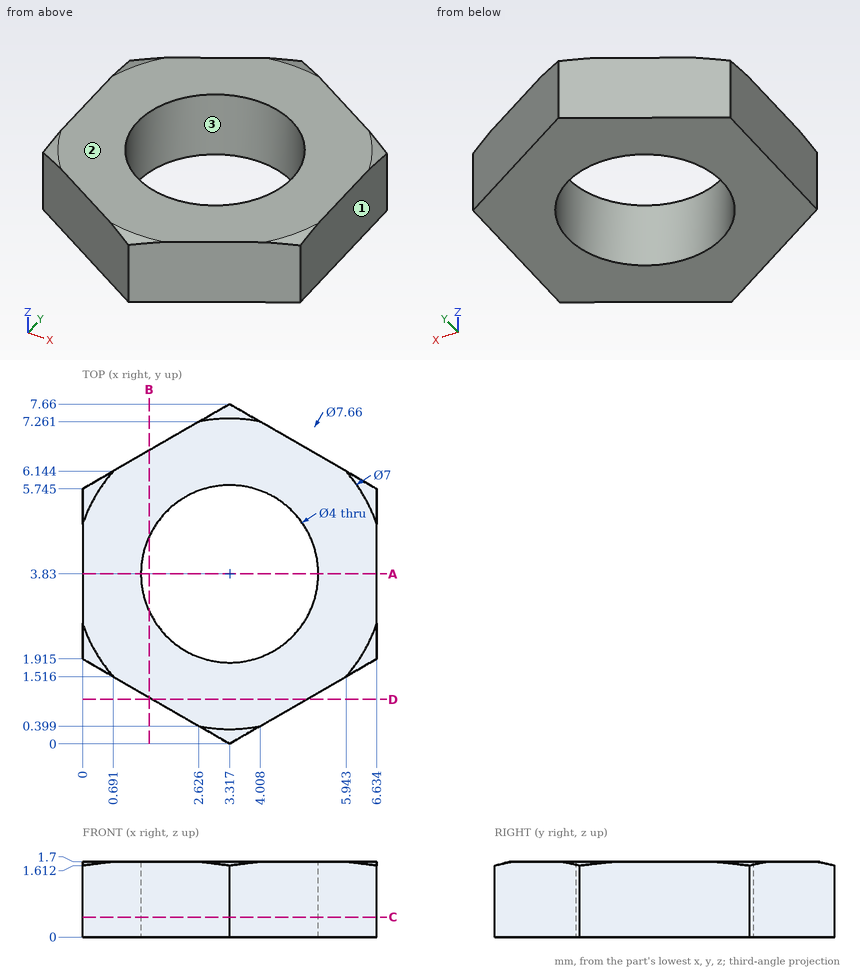
Part print with two shaded views. Sizes in mm from the minimum x, y, z corner. Round coordinates to 2 decimals unless told otherwise and drop trailing zeros. Write each loop counter-clockwise with the first axis right and the second up, starting at its lowest first coordinate (ties: lowest second). Pieces come first, ordered by that corner, then holes. Notation, with made-up numbers: M -12,-38 L 16,-38 A20 cw 16,-31 Z; hole C 43,24.25 d9. An arc over 180 degrees is marked long. Use CSV: the item, a comma, the result in double quotes.
1. Two-plate mould, pull along X, no slides. Class the marked faces 1, 2 and 3: +X half, -X half, draft (parallel to the pull), parting line (faces both ways), or undercut.
Reply:
face 1,"+X half"
face 2,"draft"
face 3,"undercut"
2. Flat gauge pin, fed straight in: pin 1 (3 mm diameter, centred on x = 3.32, y = 3.83, fed in from +Z). Where does the tip first touch, or does it go through?
Reply:
pin 1,"passes through"
3. Saw through at B-B (x = 1.5). Give the cut face in (y, z).
Reply:
outline,"M 1.05,0 L 2.99,0 L 2.99,1.7 L 1.05,1.7 Z; M 4.67,0 L 6.61,0 L 6.61,1.7 L 4.67,1.7 Z"
4. Wall check: probe 1 along Y at (x, z) = (2.75, 1.5); probe 2 along X at (y, z) = (3.5, 0.8) (1 decimal); probe 3 along X at (y, z) = (5, 1.15) (1 decimal). Give the ranges that are in metal, low to high. Write a range as from..to.
Reply:
probe 1,"y = 0.33..1.91, 5.75..7.33"
probe 2,"x = 0..1.3, 5.3..6.6"
probe 3,"x = 0..1.7, 4.9..6.6"
5. Saw through at A-A (y = 3.83). Give the cut face in (x, z).
Reply:
outline,"M 0,0 L 1.32,0 L 1.32,1.7 L 0,1.7 Z; M 5.32,0 L 6.63,0 L 6.63,1.7 L 5.32,1.7 Z"
6. Saw through at D-D (y = 1). Give the cut face in (x, z) (1 decimal).
Reply:
outline,"M 1.6,0 L 5,0 L 5,1.7 L 1.6,1.7 Z"
7. Saw through at C-C (z = 0.45). Give the cut face in (x, y) (1 decimal).
Reply:
outline,"M 0,1.9 L 3.3,0 L 6.6,1.9 L 6.6,5.7 L 3.3,7.7 L 0,5.7 Z; hole C 3.3,3.8 d4"
